from build123d import *

# Parameters (mm, degrees)
SKETCH1_W           = 60
SKETCH1_H           = 60
BOSS_EXTRUDE1_DEPTH = 5
SKETCH2_R           = 5
CUT_EXTRUDE1_DEPTH  = 43.720018727
BOSS_EXTRUDE2_DEPTH = 5
SKETCH4_R           = 1.75
CUT_EXTRUDE2_DEPTH  = 57.789083467
FILLET1_R           = 20
SKETCH8_R           = 2.1
SKETCH8_R_2         = 0.5
CUT_EXTRUDE3_DEPTH  = 10


with BuildPart() as part:
    # Sketch1 → Boss-Extrude1 (new body)
    with BuildSketch(Plane(origin=(0, 0, 0), x_dir=(1, 0, 0), z_dir=(0, 1, 0))):
        Rectangle(SKETCH1_W, SKETCH1_H)
    extrude(amount=BOSS_EXTRUDE1_DEPTH)

    # Sketch2 → Cut-Extrude1 (cut, through all)
    with BuildSketch(Plane(origin=(0, 5, 0), x_dir=(1, 0, 0), z_dir=(0, 1, 0))):
        with Locations(Location((0, 0, 0), (0, 0, 270))):
            Circle(SKETCH2_R)
    extrude(amount=-CUT_EXTRUDE1_DEPTH, mode=Mode.SUBTRACT)

    # Sketch3 → Cut-Revolve1 (revolve, cut)
    with BuildSketch(Plane.XY):
        with BuildLine():
            Line((0, 2.007275927), (0, 240.687318419))
            ThreePointArc((0, 240.687318419), (119.340021246, 121.347297173), (0, 2.007275927))
        make_face()
    revolve(axis=Axis((0, 2.007275927, 0), (0, 1, 0)), mode=Mode.SUBTRACT)

    # Sketch5 → Boss-Extrude2 (add)
    with BuildSketch(Plane(origin=(0, 0, 0), x_dir=(1, 0, 0), z_dir=(0, 1, 0))):
        Polygon((-30, -30), (-40, -30), (-40, 40), (30, 40), (30, 30), (-30, 30), align=None)
    extrude(amount=BOSS_EXTRUDE2_DEPTH)

    # Sketch4 → Cut-Extrude2 (cut, through all)
    with BuildSketch(Plane(origin=(0, 5, 0), x_dir=(1, 0, 0), z_dir=(0, 1, 0))):
        with Locations(Location((-32.627416998, 10, 0), (0, 0, 270))):
            Circle(SKETCH4_R)
        with Locations(Location((-10, 32.627416998, 0), (0, 0, 270))):
            Circle(SKETCH4_R)
        with Locations(Location((11, 32.627416998, 0), (0, 0, 270))):
            Circle(SKETCH4_R)
        with Locations(Location((-32.627416998, -11, 0), (0, 0, 270))):
            Circle(SKETCH4_R)
    extrude(amount=-CUT_EXTRUDE2_DEPTH, mode=Mode.SUBTRACT)

    # Fillet1
    fillet1_edges = [part.edges().sort_by_distance(p)[0] for p in [
        (30, 2.5, -40),
        (-40, 2.5, -40),
        (-40, 2.5, 30),
        (30, 2.5, 30),
    ]]
    fillet(fillet1_edges, radius=FILLET1_R)

    # Sketch8 → Cut-Extrude3 (cut)
    with BuildSketch(Plane(origin=(0, 5, 0), x_dir=(1, 0, 0), z_dir=(0, 1, 0))):
        with Locations(Location((-30.428243041, 30.737374818, 0), (0, 0, 270))):
            Circle(SKETCH8_R)
        with Locations(Location((-20.428243041, 30.737374818, 0), (0, 0, 270))):
            Circle(SKETCH8_R_2)
        with Locations(Location((-30.428243041, 20.737374818, 0), (0, 0, 270))):
            Circle(SKETCH8_R_2)
    extrude(amount=-CUT_EXTRUDE3_DEPTH, mode=Mode.SUBTRACT)


solid = part.part
CAD build for the part. Positions are in the model's coordinates, mm. Round coordinates to 2 decimals unless told otherwise and drop trailing zeros. Write each loop counter-clockwise with the first axis right and the second up, starting at its lowest first coordinate (ties: lowest second). Pieces come first, ordered by that corner, then holes.
(1) Slice it at C-C, the plane y = 1.35. Count the separate pieces of the cut face and the enclosed holes in it, and give its area (3 significant figures).
(2) Slice it at B-B, the plane z = 0. Write the cut outline in (x, y), and give its area (3 significant figures).
(3) Slice it at D-D, the plane x = 23. Write the cut outline in (y, z), and give its area (3 significant figures).
(4) Probe line 1 along X through (y, z) = (1.5, -10); line 2 along X through (y, z) = (2.1, -32.5); line 3 along Z through (x, y) = (-2.5, 0.2). List the from-to ranges inside material, lowest first.
(5) Mould opens along X. For faces 1 (the face through (30, 2, -5)), 2 (the face through (-34.297, 2.535, -33.986)), 3 (the face through (-8.8, 2.5, -33.9)), 4 (the face through (-5, 2, 30)) say: pulls with the +X half, pulls with the -X half, needs draft (parallel to the pull), parting line crosses it, or undercut.
(6) Slice it at A-A, the plane x = 0. Write the cut outline in (y, z), and give its area (3 significant figures).
From the geometry:
1. separate pieces: 1
1. enclosed holes: 8
1. area: 4,420 mm2
2. outline: (-40, 0) - (-5, 0) - (-5, 2.11) arc R119.34 cw to (-26.56, 5) - (-40, 5) - close; (5, 0) - (30, 0) - (30, 5) - (26.56, 5) arc R119.34 cw to (5, 2.11) - close
2. area: 223 mm2
3. outline: (0, -35.2) - (5, -35.2) - (5, -13.28) arc R117.1 cw to (5, 13.28) - (5, 25.2) - (0, 25.2) - close
3. area: 289 mm2
4. line 1: x = -40 to -34.38, -30.88 to 30
4. line 2: x = -35.61 to -31.57, -29.29 to -11.75, -8.25 to 9.25, 12.75 to 25.61
4. line 3: z = -40 to -4.33, 4.33 to 30
5. face 1: pulls with the +X half
5. face 2: pulls with the -X half
5. face 3: undercut
5. face 4: needs draft
6. outline: (0, -40) - (5, -40) - (5, -26.56) arc R119.34 cw to (2.11, -5) - (0, -5) - close; (0, 5) - (2.11, 5) arc R119.34 cw to (5, 26.56) - (5, 30) - (0, 30) - close
6. area: 223 mm2
